Read the model definition and answer for the solid it produces. Units are mm, in the model's axes. Face numbers are marked on the shaded views. A direction names the side the tool comes from. Coordinates: 2 decimals unless noted, no trailing zeros. Order: outer loops, then holes, each group sorted by start corner. A loop starts at its lowest first (then second) coordinate and runs counter-clockwise, first axis right, second up. Notation, with made-up numbers: (47, -18) - (59, -18) arc R15 cw to (59, -12) - close; hole circle Ø6 at (5.5, 60). An arc over 180 degrees is marked (long way). Answer as a JSON object with one key per item and string values. Group by question number.
Autodesk Inventor part; units mm, degrees
ref_plane "YZ Plane" through (0, 0, 0) normal (1, 0, 0) x (0, 1, 0)
ref_plane "XZ Plane" through (0, 0, 0) normal (0, 1, 0) x (-1, 0, 0)
ref_plane "XY Plane" through (0, 0, 0) normal (0, 0, 1) x (1, 0, 0)
sketch "Sketch1" plane through (0, 0, 0) normal (0, 1, 0) x (-1, 0, 0)
  circle A0 centre (0, 0) radius 15
  dimension "d0" = 30
extrude "Extrusion1" add sketch "Sketch1" along normal blind 20
sketch "Sketch2" plane through (0, 20, 0) normal (0, 1, 0) x (1, 0, 0)
  circle A0 centre (0, 0) radius 17.5
  dimension "d3" = 35
extrude "Extrusion2" add sketch "Sketch2" along normal blind 25
sketch "Sketch3" plane through (0, 45, 0) normal (0, 1, 0) x (1, 0, 0)
  circle A0 centre (0, 0) radius 7.5
  dimension "d6" = 15
extrude "Extrusion3" add sketch "Sketch3" along normal blind 10
sketch "Sketch4" plane through (0, 55, 0) normal (0, 1, 0) x (1, 0, 0)
  circle A0 centre (0, 0) radius 2.5
  dimension "d9" = 5
extrude "Extrusion4" add sketch "Sketch4" along normal blind 20
sketch "Sketch5" plane through (0, 0, 0) normal (1, 0, 0) x (0, 1, 0)
  circle A0 centre (70, 0) radius 1
  point P0 (0, 0)
  dimension "d12" = 2
extrude "Extrusion5" cut sketch "Sketch5" along normal mid plane 10
properties part number "trail 8" material "Iron, Malleable"
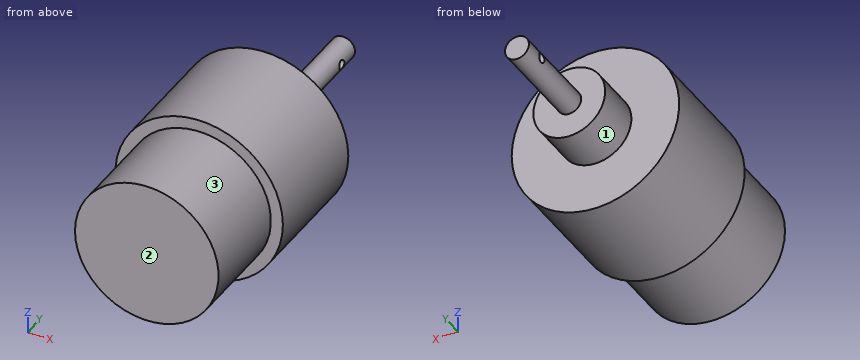
1. Given pin 1 (2 mm diameter, centred on x = 8.5, z = 12, fed in from +Y); pin 2 (1.5 mm diameter, centred on y = 30, z = -8.5, fed in from +X); pin 3 (6 mm diameter, centred on y = 11.5, z = 10, fed in from -X), each flat-ended and moving along its own axis, determine where each tip first touches the part or whether it passes through.
2. A cutting plane is placed at B-B on x = 0. Write down the section's boundary in (y, z).
3. A cutting plane is placed at A-A on z = 0. Write down the section's boundary in (x, y), and give its area (4 significant figures).
4. Straight lines are drawn through the part: L1, parallel to Y at x = -1.4, z = 0; L2, parallel to Z at x = 0, y = 70; L3, parallel to Y at x = 9, z = -11. For each, find the intervals that lie inside material, in ascending order.
5. A cutting plane is placed at C-C on y = 30.5. Write down the section's boundary in (x, z).
6. A cutting plane is placed at D-D on x = 13.5. Write down the section's boundary in (y, z), and give its area (3 significant figures).
7. For the marked faces 1, 2 and 3, determine the directions among +Z, -Z, +X, -X, +Y, -Y from which every point of the face is accessible in a straight line to the end or side of a thin tool.
Derived:
{
 "1": {"pin 1": "stops at y = 45", "pin 2": "stops at x = 15.69", "pin 3": "stops at x = -13.27"},
 "2": {"outline": "(0, -15) - (20, -15) - (20, -17.5) - (45, -17.5) - (45, -7.5) - (55, -7.5) - (55, -2.5) - (75, -2.5) - (75, 2.5) - (55, 2.5) - (55, 7.5) - (45, 7.5) - (45, 17.5) - (20, 17.5) - (20, 15) - (0, 15) - close; hole circle Ø2 at (70, 0)"},
 "3": {"outline": "(-17.5, 20) - (-15, 20) - (-15, 0) - (15, 0) - (15, 20) - (17.5, 20) - (17.5, 45) - (7.5, 45) - (7.5, 55) - (2.5, 55) - (2.5, 69) - (-2.5, 69) - (-2.5, 55) - (-7.5, 55) - (-7.5, 45) - (-17.5, 45) - close; (-2.5, 71) - (2.5, 71) - (2.5, 75) - (-2.5, 75) - close", "area": "1,715 mm2"},
 "4": {"L1": "y = 0 to 69, 71 to 75", "L2": "z = -2.5 to -1, 1 to 2.5", "L3": "y = 0 to 45"},
 "5": {"outline": "circle Ø35 at (0, 0)"},
 "6": {"outline": "(0, -6.54) - (20, -6.54) - (20, -11.14) - (45, -11.14) - (45, 11.14) - (20, 11.14) - (20, 6.54) - (0, 6.54) - close", "area": "818 mm2"},
 "7": {"face 1": "+Y", "face 2": "+Z, -Z, +X, -X, -Y", "face 3": "-Y"}
}
